The listing builds one solid part. Answer for the finished solid, in the listing's coordinates (mm). Face numbers are marked on the shaded views. A direction names the side the tool comes from. Coordinates: 2 decimals unless noted, no trailing zeros. Write each loop counter-clockwise with the first axis right and the second up, starting at its lowest first coordinate (ties: lowest second). Pieces come first, ordered by that corner, then holes.
```python
from build123d import *

# Parameters (mm, degrees)
SKETCH_2_R             = 7.94
EXTRUDE_1_DEPTH        = 7.875
EXTRUDE_1_2_DEPTH      = 7.875
EXTRUDE_2_DEPTH        = 3.43
PATTERN_LINEAR_1_COUNT = 3
PATTERN_LINEAR_1_PITCH = 29.29
EXTRUDE_3_DEPTH        = 75.24
EXTRUDE_3_DEPTH_BACK   = 16.66
SKETCH_4_R             = 3.97
CHAMFER_1_SIZE         = 0.686


with BuildPart() as part:
    # Sketch 2 → Extrude 1 (new, symmetric)
    with BuildSketch(Plane.XY):
        with Locations((12.7, 0)):
            Circle(SKETCH_2_R)
    extrude(amount=EXTRUDE_1_DEPTH, both=True)



with BuildPart() as body_2:
    # Sketch 2 → Extrude 1 2 (new, symmetric)
    with BuildSketch(Plane.XY):
        with Locations((-12.7, 0)):
            Circle(SKETCH_2_R)
    extrude(amount=EXTRUDE_1_2_DEPTH, both=True)


with BuildPart() as part_1:
    add(part.part)

    add(body_2.part)  # Extrude 2 merges body 2
    # Sketch 3 → Extrude 2 (add)
    with BuildSketch(Plane.XY.offset(7.875)):
        with BuildLine():
            ThreePointArc((-10.428153415, 11.849174574), (-24.765, 0), (-10.428153415, -11.849174574))
            ThreePointArc((-10.428153415, -11.849174574), (0, -10.8585), (10.428153415, -11.849174574))
            ThreePointArc((10.428153415, -11.849174574), (24.765, 0), (10.428153415, 11.849174574))
            ThreePointArc((10.428153415, 11.849174574), (0, 10.8585), (-10.428153415, 11.849174574))
        make_face()
    extrude_2 = extrude(amount=EXTRUDE_2_DEPTH)

    # Mirror 1: Extrude 2 across plane
    add(extrude_2.mirror(Plane.XY))


with BuildPart() as pattern_linear_1_1:
    # Pattern Linear 1: pattern copy
    add(part_1.part.moved(Location(Vector(0, 0, 1) * (1 * PATTERN_LINEAR_1_PITCH))))


with BuildPart() as pattern_linear_1_2:
    # Pattern Linear 1: pattern copy
    add(part_1.part.moved(Location(Vector(0, 0, 1) * (2 * PATTERN_LINEAR_1_PITCH))))


with BuildPart() as part_2:
    add(part_1.part)

    add(pattern_linear_1_1.part)  # Extrude 3 merges Pattern Linear 1_1

    add(pattern_linear_1_2.part)  # Extrude 3 merges Pattern Linear 1_2
    # Sketch 4 → Extrude 3 (add, two sides: drawn at the far end of the back side and taken through both)
    with BuildSketch(Plane.XY.offset(-EXTRUDE_3_DEPTH_BACK)):
        with Locations(Location((12.7, 0, 0), (0, 0, 180))):
            Circle(SKETCH_4_R)
        with Locations(Location((-12.7, 0, 0), (0, 0, 180))):
            Circle(SKETCH_4_R)
    extrude(amount=EXTRUDE_3_DEPTH + EXTRUDE_3_DEPTH_BACK)

    # Chamfer 1
    chamfer_1_edges = [part_2.edges().sort_by_distance(p)[0] for p in [
        (16.67, 0, -16.66),
        (16.67, 0, 75.24),
        (-8.73, 0, -16.66),
        (-8.73, 0, 75.24),
    ]]
    chamfer(chamfer_1_edges, length=CHAMFER_1_SIZE)


solid = part_2.part
```
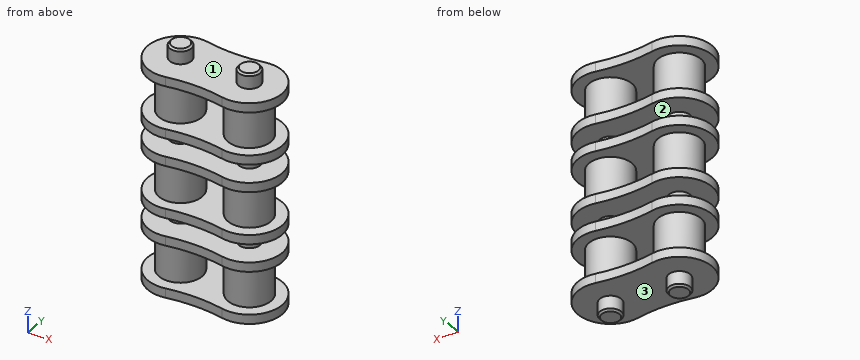
(1) Find the intervals of material crossed by probe 1 along Z at (x, y) = (19, -9.5) (3 decimals); probe 2 along Z at (x, y) = (-13, -5.5) (3 decimals); probe 3 along X at (y, z) = (-4.5, 27), in increasing order.
(2) Which of the six approach directions +Z, -Z, +X, -X, +Y, -Y give full straight-line access (tool end or side, diameter ignored) to the marked faces 1, 2 and 3?
(3) Each of these flat-tipped pins is pushed along its axis until it touches: pin 1 (3 mm diameter, centred on y = 9.5, z = 36, fed in from -X); pin 2 (12 mm diameter, centred on x = 1, y = 5.5, fed in from -Z) (3 decimals); pin 3 (5 mm diameter, centred on y = 6, z = 66, fed in from +X). Where does it stop, or does it pass through?
(4) Section D-D, the plane y = 0 is taken. State how many separate pieces and enclosed holes the cut face has, plus the area to 3 significant figures.
(5) Section C-C, the plane z = 42 is taken. Write down the section's boundary in (x, y).
(6) Section A-A, the plane y = -10 is taken. Write down the section's boundary in (x, z) (3 decimals), plus the area to 3 significant figures.
(7) Section B-B, the plane x = 21.5 is taken. Write down the section's boundary in (y, z) (3 decimals).
Solution:
1. probe 1: z = -11.305 to -7.875, 7.875 to 11.305, 17.985 to 21.415, 37.165 to 40.595, 47.275 to 50.705, 66.455 to 69.885
1. probe 2: z = -11.305 to 11.305, 17.985 to 40.595, 47.275 to 69.885
1. probe 3: x = -19.24 to -6.16, 6.16 to 19.24
2. face 1: +Z
2. face 2: none
2. face 3: -Z
3. pin 1: stops at x = -21.21
3. pin 2: stops at z = -11.305
3. pin 3: stops at x = 24.23
4. separate pieces: 1
4. enclosed holes: 5
4. area: 2,900 mm2
5. outline: circle Ø7.94 at (-12.7, 0); circle Ø7.94 at (12.7, 0)
6. outline: (-19.45, -11.305) - (19.45, -11.305) - (19.45, -7.875) - (-19.45, -7.875) - close; (-19.45, 7.875) - (19.45, 7.875) - (19.45, 11.305) - (-19.45, 11.305) - close; (-19.45, 17.985) - (19.45, 17.985) - (19.45, 21.415) - (-19.45, 21.415) - close; (-19.45, 37.165) - (19.45, 37.165) - (19.45, 40.595) - (-19.45, 40.595) - close; (-19.45, 47.275) - (19.45, 47.275) - (19.45, 50.705) - (-19.45, 50.705) - close; (-19.45, 66.455) - (19.45, 66.455) - (19.45, 69.885) - (-19.45, 69.885) - close
6. area: 801 mm2
7. outline: (-8.254, -11.305) - (8.254, -11.305) - (8.254, -7.875) - (-8.254, -7.875) - close; (-8.254, 7.875) - (8.254, 7.875) - (8.254, 11.305) - (-8.254, 11.305) - close; (-8.254, 17.985) - (8.254, 17.985) - (8.254, 21.415) - (-8.254, 21.415) - close; (-8.254, 37.165) - (8.254, 37.165) - (8.254, 40.595) - (-8.254, 40.595) - close; (-8.254, 47.275) - (8.254, 47.275) - (8.254, 50.705) - (-8.254, 50.705) - close; (-8.254, 66.455) - (8.254, 66.455) - (8.254, 69.885) - (-8.254, 69.885) - close
